Part model, mm, in its own coordinate system. A direction names the side the tool comes from. Give positions to 0.01 mm unless a question says otherwise; leave off trailing zeros. Write each loop counter-clockwise with the first axis right and the second up, starting at its lowest first coordinate (ties: lowest second). Pieces come first, ordered by that corner, then holes.
from build123d import *

# Parameters (mm, degrees)
SKETCH_1_W          = 8.5
SKETCH_1_H          = 25.5
EXTRUDE_1_DEPTH     = 5
EXTRUDE_2_DEPTH     = 5
SKETCH_3_W          = 8.5
SKETCH_3_H          = 25.5
EXTRUDE_3_DEPTH     = 5
EXTRUDE_4_DEPTH     = 25.5
EXTRUDE_5_DEPTH     = 35.5
CUT_EXTRUDE_1_DEPTH = 5
CUT_EXTRUDE_2_DEPTH = 25.5
EXTRUDE_6_REACH     = 63.804
SKETCH_8_W          = 22
SKETCH_8_H          = 4
EXTRUDE_7_DEPTH     = 4
SKETCH_10_W         = 26
SKETCH_10_H         = 34
CUT_EXTRUDE_3_DEPTH = 4


with BuildPart() as part:
    # 草图1 → 凸台-拉伸1 (new body)
    with BuildSketch(Plane.XY):
        Polygon((-16.963203436, -12.75), (4.25, -33.963203436), (25.463203436, -12.75), (4.25, 8.463203436), align=None)
        with Locations((4.25, -12.75)):
            Rectangle(SKETCH_1_W, SKETCH_1_H, mode=Mode.SUBTRACT)
    extrude(amount=EXTRUDE_1_DEPTH)

    # 草图2 → 凸台-拉伸2 (add)
    with BuildSketch(Plane.XY.offset(5)):
        Polygon((1.25, 0), (1.25, 5.463203436), (-16.963203436, -12.75), (4.25, -33.963203436), (25.463203436, -12.75), (7.25, 5.463203436), (7.25, 0), (8.5, 0), (8.5, -25.5), (0, -25.5), (0, 0), align=None)
    extrude(amount=EXTRUDE_2_DEPTH)

    # 草图3 → 凸台-拉伸3 (add)
    with BuildSketch(Plane.XY.offset(5)):
        with Locations((4.25, -12.75)):
            Rectangle(SKETCH_3_W, SKETCH_3_H)
    extrude(amount=-EXTRUDE_3_DEPTH)

    # 草图4 → 凸台-拉伸4 (add)
    with BuildSketch(Plane(origin=(0, 0, 0), x_dir=(-1, 0, 0), z_dir=(0, 0, -1))):
        Polygon((-25.463203436, -12.75), (-4.25, -33.963203436), (16.963203436, -12.75), (-4.25, 8.463203436), align=None)
        Polygon((12.720562748, -12.75), (-4.25, 4.220562748), (-21.220562748, -12.75), (-4.25, -29.720562748), align=None, mode=Mode.SUBTRACT)
    extrude(amount=EXTRUDE_4_DEPTH)

    # 草图5 → 凸台-拉伸5 (add)
    with BuildSketch(Plane.XY.offset(10)):
        Polygon((4.25, 8.463203436), (25.463203436, -12.75), (28.998737342, -9.214466094), (7.785533906, 11.998737342), align=None)
        Polygon((-16.963203436, -12.75), (-20.498737342, -16.285533906), (0.714466094, -37.498737342), (4.25, -33.963203436), align=None)
    extrude(amount=-EXTRUDE_5_DEPTH)

    # 草图6 → 切除-拉伸1 (cut)
    with BuildSketch(Plane.XY.offset(10)):
        Polygon((7.25, 5.463203436), (10.785533906, 8.998737342), (7.785533906, 11.998737342), (4.25, 8.463203436), align=None)
    extrude(amount=-CUT_EXTRUDE_1_DEPTH, mode=Mode.SUBTRACT)

    # 草图7 → 切除-拉伸2 (cut)
    with BuildSketch(Plane(origin=(0, 0, -25.5), x_dir=(-1, 0, 0), z_dir=(0, 0, -1))):
        Polygon((-4.25, 4.220562748), (-7.785533906, 7.756096654), (-24.756096654, -9.214466094), (-21.220562748, -12.75), align=None)
        Polygon((12.720562748, -12.75), (16.256096654, -16.285533906), (-0.714466094, -33.256096654), (-4.25, -29.720562748), align=None)
    extrude(amount=-CUT_EXTRUDE_2_DEPTH, mode=Mode.SUBTRACT)

    # 凸台-拉伸6: up to this face of the body (flat: up to its plane)
    extrude_6_end = Plane(part.part.faces().sort_by_distance((-9.892135624, -26.892135624, -7.75))[0])
    # 草图8 → 凸台-拉伸6 (add, up to the picked face)
    with BuildSketch(Plane(origin=(9.892135624, 9.892135624, 0), x_dir=(0, 0, -1), z_dir=(0.7071067811865537, 0.7071067811865415, 0)), mode=Mode.PRIVATE) as extrude_6_sk1:
        with Locations((36.5, -11.52081528)):
            Rectangle(SKETCH_8_W, SKETCH_8_H)
    extrude_6_tool1 = split(extrude(extrude_6_sk1.sketch, amount=-EXTRUDE_6_REACH, mode=Mode.PRIVATE), bisect_by=extrude_6_end, keep=Keep.BOTH, mode=Mode.PRIVATE)
    add(extrude_6_tool1.solids().sort_by(Axis((18.038582, 1.745689, -36.5), (-0.7071067811865537, -0.7071067811865415, 0)))[0])

    # 草图9 → 凸台-拉伸7 (add)
    with BuildSketch(Plane(origin=(0, 0, -47.5), x_dir=(-1, 0, 0), z_dir=(0, 0, -1))):
        Polygon((-16.624368671, 3.159902577), (-28.998737342, -9.214466094), (-0.714466094, -37.498737342), (11.659902577, -25.124368671), align=None)
    extrude(amount=EXTRUDE_7_DEPTH)

    # 草图10 → 切除-拉伸3 (cut)
    with BuildSketch(Plane(origin=(9.560660172, -9.560660172, 0), x_dir=(0, 0, -1), z_dir=(0.7071067811865416, -0.7071067811865536, 0))):
        with Locations((38.5, -6.01040764)):
            Rectangle(SKETCH_10_W, SKETCH_10_H)
    extrude(amount=-CUT_EXTRUDE_3_DEPTH, mode=Mode.SUBTRACT)


solid = part.part
1) Mould opens along X. For faces 6 (the flat face through (18.41, -0.71, -36.35)), 7 (the flat face through (-7.65, -24.89, -19.67)), 8 (the flat face through (-6.159, -1.945, -7.502)), 9 (the flat face through (-5, -4, -25.5)) say: +X half, -X half, draft (parallel to the pull), parting line (faces both ways), or undercut.
Check result:
face 6: +X half
face 7: undercut
face 8: -X half
face 9: draft
2) Saw through at B-B (y = -24). Write the cut outline in (x, z).
Check result:
outline: (-12.78, -25.5) - (-10.54, -25.5) - (-10.54, -51.5) - (-8.54, -51.5) - (-8.54, 0) - (9.97, 0) - (9.97, -25.5) - (14.21, -25.5) - (14.21, 10) - (8.5, 10) - (8.5, 5) - (0, 5) - (0, 10) - (-12.78, 10) - close; (-4.88, -51.5) - (14.21, -51.5) - (14.21, -47.5) - (-4.88, -47.5) - close
3) 3-axis set-ups, long thin cutter, end or side, ignore diameter. For faces 1 (the flat face through (15.549, 2.084, -38.318)), 2 (the flat face through (0, -13, 7)), 3 (the flat face through (4, -12, 0)), 4 (the flat face through (8.993, 7.206, 7.535)), 5 (the flat face through (-7.76, -26.88, -36.35)): which of +Z, -Z, +X, -X, +Y, -Y reach the whole face in a straight line?
Check result:
face 1: -Z, -X, +Y
face 2: +Z
face 3: none
face 4: +Z, -X, +Y
face 5: +X, -Y
4) Saw through at D-D (z = -16.5). Write the cut outline in (x, y), and give its area (3 significant figures).
Check result:
outline: (-20.5, -16.29) - (0.71, -37.5) - (29, -9.21) - (7.79, 12) - close; hole (-16.26, -16.29) - (0.71, -33.26) - (24.76, -9.21) - (7.79, 7.76) - close
area: 384 mm2
5) Saw through at A-A (z = -38.5). Write the cut outline in (x, y).
Check result:
outline: (-11.66, -25.12) - (-8.83, -27.95) - (-6.71, -25.83) - (-9.54, -23) - close; (14.5, 1.04) - (17.33, -1.79) - (19.45, 0.33) - (16.62, 3.16) - close
6) Saw through at C-C (x = 5.5). Write the cut outline in (y, z), and give its area (3 significant figures).
Check result:
outline: (-32.71, -51.5) - (-13.62, -51.5) - (-13.62, -47.5) - (-32.71, -47.5) - close; (-32.71, -25.5) - (-28.47, -25.5) - (-28.47, 0) - (5.47, 0) - (5.47, -25.5) - (9.71, -25.5) - (9.71, 5) - (-25.5, 5) - (-25.5, 10) - (-32.71, 10) - close
area: 541 mm2
7) Drill centre lines: L1, parallel to Z at x = -5, y = -27; L2, parallel to Z at x = -10, y = -17; L3, parallel to X at y = -12.5, z = -11.5. Where is each one in solid material? Low to high.
Check result:
L1: z = -51.5 to -47.5, 0 to 10
L2: z = 0 to 10
L3: x = -16.71 to -12.47, 21.47 to 25.71
8) Flat gauge pins, fed straight in: P1, Ø2, axis at y = -2, z = -2, coming from the -X side; P2, Ø5.5, axis at y = -18, z = 6.5, coming from the +X side; P3, Ø6, axis at x = 1, z = -12, coming from the -Y side; P4, Ø1.5, axis at x = 14.5, y = 6.5, coming from the +Z side. Where does each tip first touch, or does it go through?
Check result:
P1: stops at x = -7.21
P2: stops at x = 22.96
P3: stops at y = -37.5
P4: passes through
